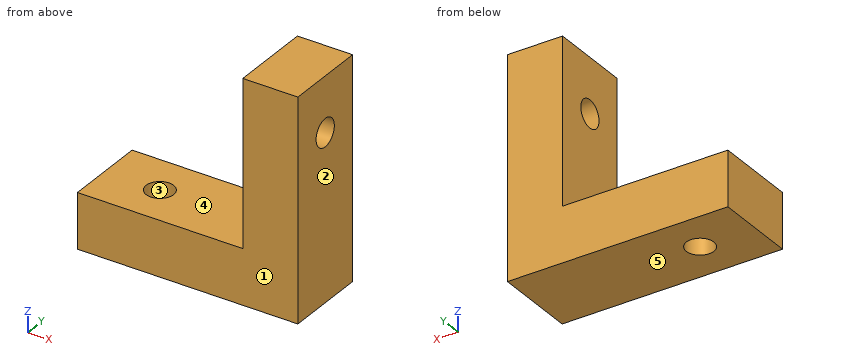
from build123d import *

# Parameters (mm, degrees)
SKETCH1_R           = 5
BOSS_EXTRUDE1_DEPTH = 20
SKETCH2_W           = 20
SKETCH2_H           = 30
BOSS_EXTRUDE2_DEPTH = 60
SKETCH3_R           = 5
CUT_EXTRUDE1_DEPTH  = 60


with BuildPart() as part:
    # Sketch1 → Boss-Extrude1 (new body)
    with BuildSketch(Plane.XY):
        Polygon((-20, 15), (-40, 15), (-40, -15), (40, -15), (40, 15), align=None)
        with Locations((-20, 0)):
            Circle(SKETCH1_R, mode=Mode.SUBTRACT)
    extrude(amount=BOSS_EXTRUDE1_DEPTH)

    # Sketch2 → Boss-Extrude2 (add)
    with BuildSketch(Plane.XY.offset(20)):
        with Locations((30, 0)):
            Rectangle(SKETCH2_W, SKETCH2_H)
    extrude(amount=BOSS_EXTRUDE2_DEPTH)

    # Sketch3 → Cut-Extrude1 (cut)
    with BuildSketch(Plane.ZY.offset(-20)):
        with Locations(Location((60, 0, 0), (0, 0, 270))):
            Circle(SKETCH3_R)
    extrude(amount=-CUT_EXTRUDE1_DEPTH, mode=Mode.SUBTRACT)


solid = part.part
CAD build for the part. Positions are in the model's coordinates, mm. Face numbers are marked on the shaded views. A direction names the side the tool comes from. Coordinates: 2 decimals unless noted, no trailing zeros. Write each loop counter-clockwise with the first axis right and the second up, starting at its lowest first coordinate (ties: lowest second). Pieces come first, ordered by that corner, then holes. Notation, with made-up numbers: M 79.5,52.25 L 112.5,52.25 A25 ccw 112.5,70.25 Z; hole C -12,-35 d6. An arc over 180 degrees is marked long. Answer as a JSON object with one key per item and string values. Group by question number.
1) Wall check: line 1 (Y direction, x = -20, z = 15); line 2 (X direction, y = 4.75, z = 49); line 3 (Z direction, x = -17, y = -4.25). Give the ranges that are in metal, low to high. Write a range as from..to.
2) Mould opens along X. For the marked faces 1, 2 and 3 say: +X half, -X half, draft (parallel to the pull), parting line (faces both ways), or undercut.
3) Saw through at B-B (z = 60). Write the cut outline in (x, y), plus the area to 3 significant figures.
4) Tool access for the marked faces 4 and 5: list every direction of +Z, -Z, +X, -X, +Y, -Y with a clear straight run to the whole face (end or side of a thin tool).
5) Saw through at C-C (x = -20). Write the cut outline in (y, z), plus the area to 3 significant figures.
6) Saw through at A-A (y = 0). Write the cut outline in (x, z).
7) Saw through at D-D (z = 10). Write the cut outline in (x, y), plus the area to 3 significant figures.
8) Pin check, flat tips, straight feed: pin 1 Ø12 at (y, z) = (-1.5, 42.5) entering from -X; pin 2 Ø6 at (y, z) = (0, 60) entering from -X. Stop position of each tip, or through.
Values follow:
{
 "1": {"line 1": "y = -15..-5, 5..15", "line 2": "x = 20..40", "line 3": "z = 0..20"},
 "2": {"face 1": "draft", "face 2": "+X half", "face 3": "undercut"},
 "3": {"outline": "M 20,-15 L 40,-15 L 40,-5 L 20,-5 Z; M 20,5 L 40,5 L 40,15 L 20,15 Z", "area": "400 mm2"},
 "4": {"face 4": "+Z, -X, +Y, -Y", "face 5": "-Z, +X, -X, +Y, -Y"},
 "5": {"outline": "M -15,0 L -5,0 L -5,20 L -15,20 Z; M 5,0 L 15,0 L 15,20 L 5,20 Z", "area": "400 mm2"},
 "6": {"outline": "M -40,0 L -25,0 L -25,20 L -40,20 Z; M -15,0 L 40,0 L 40,55 L 20,55 L 20,20 L -15,20 Z; M 20,65 L 40,65 L 40,80 L 20,80 Z"},
 "7": {"outline": "M -40,-15 L 40,-15 L 40,15 L -40,15 Z; hole C -20,0 d10", "area": "2,320 mm2"},
 "8": {"pin 1": "stops at x = 20", "pin 2": "passes through"}
}
